Verification items for the finished model (mm, model axes). Face numbers are marked on the shaded views. A direction names the side the tool comes from. Give positions to 0.01 mm unless a question says otherwise; leave off trailing zeros. Write each loop counter-clockwise with the first axis right and the second up, starting at its lowest first coordinate (ties: lowest second). Pieces come first, ordered by that corner, then holes. Notation, with made-up numbers: (41, 66) - (49, 66) arc R18 ccw to (49, 71) - close; hole circle Ø11 at (15.25, 46). An arc over 180 degrees is marked (long way). Answer as a JSON object with one key per item and string values. Group by question number.
Item 1: Go/stop test with flat-tipped pins: pin 1 (1 mm diameter, centred on y = -5, z = 6, fed in from -X); pin 2 (5 mm diameter, centred on x = 15.5, y = -6.5, fed in from +Z); pin 3 (3 mm diameter, centred on x = 5.5, y = -3.5, fed in from -Z); pin 4 (10 mm diameter, centred on x = -14.5, z = 10, fed in from -Y). Record where each tip stops, or that it passes through.
Item 2: Scan lines: line 1 along Z through (x, y) = (-2.5, -8); line 2 along X through (y, z) = (-6.5, -4); line 3 along Z through (x, y) = (3, -8). Record each from-to range of solid material in increasing order. Write a range as [from, to].
Item 3: Tool access check on the marked faces 5, 6 and 7. Record the directions out of +Z, -Z, +X, -X, +Y, -Y that give a thin tool (end or side, any length) a straight path to the whole face; none if there is none.
Item 4: Draft check along X on the marked faces 1, 2, 3 and 4. Enter one of: +X half, -X half, draft (parallel to the pull), parting line (faces both ways), or undercut.
Item 5: Sectioned sample at A-A, the plane x = 0. Record the boundary of the cut face in (y, z) (3 decimals).
Item 6: Sectioned sample at B-B, the plane z = 10.5. Record the boundary of the cut face in (x, y) (1 decimal).
Item 7: Sectioned sample at D-D, the plane z = 17.5. Record the boundary of the cut face in (x, y) (1 decimal).
Item 8: Sectioned sample at C-C, the plane y = -1.5. Count the separate pieces of the cut face and the enclosed holes in it, and give its area (3 significant figures).
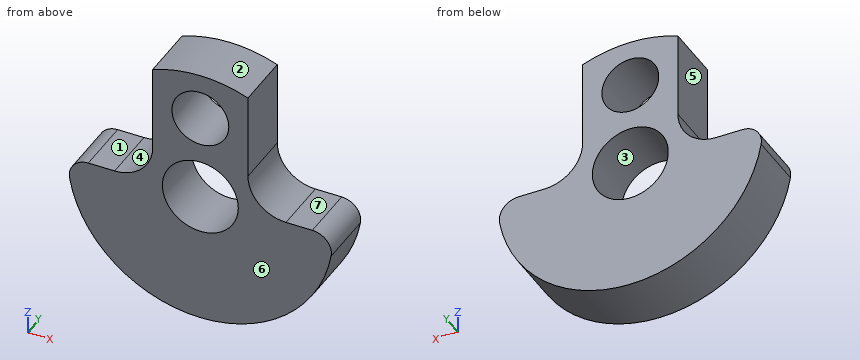
```python
from build123d import *

# Parameters (mm, degrees)
F0_R     = 6.33095
F0_R_2   = 4.74345
F1_DEPTH = 9.525
F2_R     = 6.35
F3_R     = 3.175


with BuildPart() as f1:
    # F0 (on Front) → F1 (new body)
    with BuildSketch(Plane.XZ):
        with BuildLine():
            Line((-7.9375, 0), (-22.1234, 0))
            ThreePointArc((-22.1234, 0), (0, -22.1234), (22.1234, 0))
            Line((22.1234, 0), (7.9375, 0))
            Line((7.9375, 0), (7.9375, 20.650446))
            ThreePointArc((7.9375, 20.650446), (0, 22.1234), (-7.9375, 20.650446))
            Line((-7.9375, 20.650446), (-7.9375, 0))
        make_face()
        Circle(F0_R, mode=Mode.SUBTRACT)
        with Locations((0, 14.3002)):
            Circle(F0_R_2, mode=Mode.SUBTRACT)
    extrude(amount=F1_DEPTH)

    # F2
    f2_edges = [f1.edges().sort_by_distance(p)[0] for p in [
        (-7.9375, -4.7625, 0),
        (7.9375, -4.7625, 0),
    ]]
    fillet(f2_edges, radius=F2_R)

    # F3
    f3_edges = [f1.edges().sort_by_distance(p)[0] for p in [
        (-22.1234, -4.7625, 0),
        (22.1234, -4.7625, 0),
    ]]
    fillet(f3_edges, radius=F3_R)


solid = f1.part
```
Geometry check:
{
 "1": {"pin 1": "x = -7.99", "pin 2": "z = 0.13", "pin 3": "z = -21.76", "pin 4": "through"},
 "2": {"line 1": "[-21.98, -5.82], [5.82, 10.27], [18.33, 21.98]", "line 2": "[-21.76, -4.91], [4.91, 21.76]", "line 3": "[-21.92, -5.58], [5.58, 10.63], [17.97, 21.92]"},
 "3": {"face 5": "+Z, -X, +Y, -Y", "face 6": "+Z, -Z, +X, -X, -Y", "face 7": "+Z, +X, +Y, -Y"},
 "4": {"face 1": "draft", "face 2": "parting line", "face 3": "undercut", "face 4": "-X half"},
 "5": {"outline": "(-9.525, -22.123) - (0, -22.123) - (0, -6.331) - (-9.525, -6.331) - close; (-9.525, 6.331) - (0, 6.331) - (0, 9.557) - (-9.525, 9.557) - close; (-9.525, 19.044) - (0, 19.044) - (0, 22.123) - (-9.525, 22.123) - close"},
 "6": {"outline": "(-7.9, -9.5) - (-2.8, -9.5) - (-2.8, 0) - (-7.9, 0) - close; (2.8, -9.5) - (7.9, -9.5) - (7.9, 0) - (2.8, 0) - close"},
 "7": {"outline": "(-7.9, -9.5) - (-3.5, -9.5) - (-3.5, 0) - (-7.9, 0) - close; (3.5, -9.5) - (7.9, -9.5) - (7.9, 0) - (3.5, 0) - close"},
 "8": {"separate pieces": "1", "enclosed holes": "2", "area": "927 mm^2"}
}
